from build123d import *

# Parameters (mm, degrees)
BOSS_EXTRUDE1_DEPTH = 254
FILLET1_R           = 12.7
SKETCH2_R           = 3.175
CUT_EXTRUDE1_DEPTH  = 12.7
CIRPATTERN2_COUNT   = 2
CIRPATTERN2_ANGLE   = 90
BOSS_EXTRUDE2_DEPTH = 279.4
FILLET2_R           = 12.7
SKETCH5_R           = 3.175
CUT_EXTRUDE2_DEPTH  = 12.7


with BuildPart() as part:
    # Sketch1 → Boss-Extrude1 (new body)
    with BuildSketch(Plane.XY):
        with BuildLine():
            Line((-9.525, -22.225), (9.525, -22.225))
            ThreePointArc((9.525, -22.225), (18.505256121, -18.505256121), (22.225, -9.525))
            Line((22.225, -9.525), (22.225, 9.525))
            ThreePointArc((22.225, 9.525), (18.505256121, 18.505256121), (9.525, 22.225))
            Line((9.525, 22.225), (-9.525, 22.225))
            ThreePointArc((-9.525, 22.225), (-18.505256121, 18.505256121), (-22.225, 9.525))
            Line((-22.225, 9.525), (-22.225, -9.525))
            ThreePointArc((-22.225, -9.525), (-18.505256121, -18.505256121), (-9.525, -22.225))
        make_face()
    extrude(amount=BOSS_EXTRUDE1_DEPTH)

    # Fillet1
    fillet1_edges = [part.edges().sort_by_distance(p)[0] for p in [
        (0, -22.225, 0),
        (-18.505256121, -18.505256121, 0),
        (-22.225, 0, 0),
        (-18.505256121, 18.505256121, 0),
        (0, 22.225, 0),
        (18.505256121, 18.505256121, 0),
        (22.225, 0, 0),
        (18.505256121, -18.505256121, 0),
    ]]
    fillet(fillet1_edges, radius=FILLET1_R)

    # Sketch2 → Cut-Extrude1 (cut)
    with BuildSketch(Plane(origin=(0, 22.225, 0), x_dir=(1, 0, 0), z_dir=(0, 1, 0))):
        with Locations(Location((0, -177.8, 0), (0, 0, 270))):  # turned: the seam where the file's is
            Circle(SKETCH2_R)
        with Locations(Location((0, -228.6, 0), (0, 0, 270))):  # turned: the seam where the file's is
            Circle(SKETCH2_R)
    cut_extrude1 = extrude(amount=-CUT_EXTRUDE1_DEPTH, mode=Mode.SUBTRACT)

    # CirPattern2: Cut-Extrude1 ×2 about axis
    cirpattern2_axis = Axis((0, 0, 1052.131449431), (0, 0, -1))
    for i in range(1, CIRPATTERN2_COUNT):
        add(cut_extrude1.rotate(cirpattern2_axis, i * CIRPATTERN2_ANGLE / (CIRPATTERN2_COUNT - 1)), mode=Mode.SUBTRACT)

    # Sketch4 → Boss-Extrude2 (add)
    with BuildSketch(Plane.XY.offset(254)):
        with BuildLine():
            Line((-9.525, -22.225), (9.525, -22.225))
            ThreePointArc((9.525, -22.225), (18.505256121, -18.505256121), (22.225, -9.525))
            Line((22.225, -9.525), (22.225, 9.525))
            ThreePointArc((22.225, 9.525), (18.505256121, 18.505256121), (9.525, 22.225))
            Line((9.525, 22.225), (-9.525, 22.225))
            ThreePointArc((-9.525, 22.225), (-18.505256121, 18.505256121), (-22.225, 9.525))
            Line((-22.225, 9.525), (-22.225, -9.525))
            ThreePointArc((-22.225, -9.525), (-18.505256121, -18.505256121), (-9.525, -22.225))
        make_face()
    extrude(amount=BOSS_EXTRUDE2_DEPTH)

    # Fillet2
    fillet2_edges = [part.edges().sort_by_distance(p)[0] for p in [
        (-18.505256121, -18.505256121, 533.4),
        (0, -22.225, 533.4),
        (18.505256121, -18.505256121, 533.4),
        (22.225, 0, 533.4),
        (18.505256121, 18.505256121, 533.4),
        (0, 22.225, 533.4),
        (-18.505256121, 18.505256121, 533.4),
        (-22.225, 0, 533.4),
    ]]
    fillet(fillet2_edges, radius=FILLET2_R)

    # Sketch5 → Cut-Extrude2 (cut)
    with BuildSketch(Plane(origin=(22.225, 0, 0), x_dir=(0, 0, -1), z_dir=(1, 0, 0))):
        with Locations((-431.8, 0)):
            Circle(SKETCH5_R)
        with Locations((-482.6, 0)):
            Circle(SKETCH5_R)
    extrude(amount=-CUT_EXTRUDE2_DEPTH, mode=Mode.SUBTRACT)


solid = part.part
The model under review builds one solid part; all positions refer to its coordinate system, in mm. Round coordinates to 2 decimals unless told otherwise and drop trailing zeros. Order: outer loops, then holes, each group sorted by start corner. A loop starts at its lowest first (then second) coordinate and runs counter-clockwise, first axis right, second up. Notation, with made-up numbers: (54.5, -18) -> (108.5, -18) arc R37 ccw to (108.5, 19) -> close; hole circle Ø6 at (29.5, 27). An arc over 180 degrees is marked (long way). Return JSON: item names as keys, results as strings.
1. For L1, parallel to Y at x = 16, z = 177.8 (3 decimals); L2, parallel to Y at x = 18, z = 430; L3, parallel to Y at x = -15.5, z = 218, list the stretches that pass through material, from the lowest coordinate up. Write a range as [from, to].
Answer block:
{"L1": "y = [-20.45, -3.175], [3.175, 20.45]", "L2": "y = [-18.98, -2.62], [2.62, 18.98]", "L3": "y = [-20.73, 20.73]"}
2. Insertion check: P1, Ø1, axis at x = 11, y = 1.5, coming from the +Z side; P2, Ø3, axis at y = -0.5, z = 433, coming from the +X side (3 decimals); P3, Ø1.5, axis at x = -11, z = 273.5, coming from the -Y side. Each pin has a flat end and moves straight along its axis. Give the tip position at first contact, or say it passes through.
Answer block:
{"P1": "stops at z = 533.36", "P2": "stops at x = 9.525", "P3": "stops at y = -22.2"}
3. Take a section at A-A (z = 186). Write out the cut boundary in (x, y) (3 decimals).
Answer block:
{"outline": "(-22.225, -9.525) arc R12.7 ccw to (-9.525, -22.225) -> (9.525, -22.225) arc R12.7 ccw to (22.225, -9.525) -> (22.225, 9.525) arc R12.7 ccw to (9.525, 22.225) -> (-9.525, 22.225) arc R12.7 ccw to (-22.225, 9.525) -> close"}
4. Take a section at B-B (x = -14.5). Write out the cut boundary in (y, z) (3 decimals).
Answer block:
{"outline": "(-21.21, 12.7) arc R11.685 ccw to (-9.525, 1.015) -> (9.525, 1.015) arc R11.685 ccw to (21.21, 12.7) -> (21.21, 520.7) arc R11.685 ccw to (9.525, 532.385) -> (-9.525, 532.385) arc R11.685 ccw to (-21.21, 520.7) -> close"}
